Can you work these out from the model? Positions are in its coordinate system, mm. Face numbers are marked on the shaded views. A direction names the side the tool comes from. Give positions to 0.01 mm unless a question says otherwise; leave off trailing zeros. Order: outer loops, then holes, each group sorted by start corner. A loop starts at its lowest first (then second) coordinate and runs counter-clockwise, first axis right, second up. Notation, with made-up numbers: (66, -38.5) -> (91, -38.5) arc R20 cw to (91, -28.5) -> close; hole circle Ø8 at (22, 63). An arc over 180 degrees is marked (long way). Answer as a JSON object with one key per item and string values.
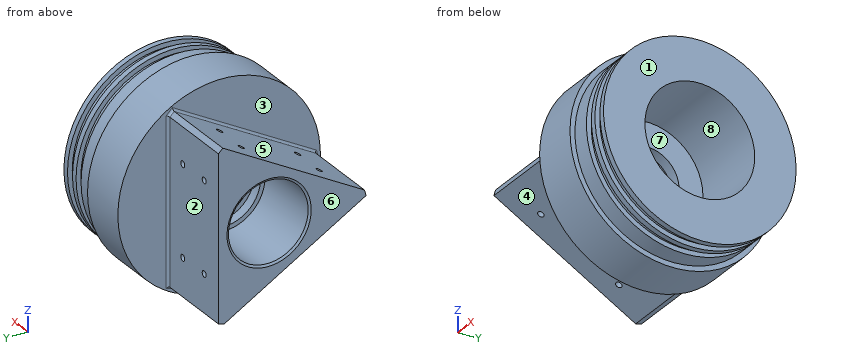
```python
from build123d import *
from OCP.BRepFilletAPI import BRepFilletAPI_MakeChamfer

# Parameters (mm, degrees)
BOSS_EXTRUDE1_DEPTH            = 22.225
SKETCH4_R                      = 22.5
CUT_EXTRUDE2_DEPTH             = 39
CHAMFER1_SIZE                  = 1.27
CHAMFER1_SIZE2                 = 0.733234842
SKETCH5_R                      = 20
CUT_EXTRUDE3_DEPTH             = 22.225
F_6_32_TAPPED_HOLE2_AT_2_COUNT = 2
F_6_32_TAPPED_HOLE2_AT_2_PITCH = 19.05
F_6_32_TAPPED_HOLE2_AT_3_COUNT = 2
F_6_32_TAPPED_HOLE2_AT_3_PITCH = 54.254423783
F_6_32_TAPPED_HOLE2_AT_4_COUNT = 2
F_6_32_TAPPED_HOLE2_AT_4_PITCH = 50.8
CIRPATTERN1_COUNT              = 3
SKETCH9_R                      = 31
CUT_EXTRUDE5_DEPTH             = 46
CUT_EXTRUDE6_REACH             = 97.461
SKETCH10_R                     = 17.5
CHAMFER2_SIZE                  = 3.81
CHAMFER2_SIZE2                 = 2.789113577
FILLET4_R                      = 1.27


with BuildPart() as part:
    # Sketch1 → Boss-Extrude1 (new, symmetric)
    with BuildSketch(Plane(origin=(0, 0, 0), x_dir=(0, 0, -1), z_dir=(1, 0, 0))):
        Polygon((-49.493351826, 28.575), (49.493351826, 28.575), (0, -57.15), align=None)
    extrude(amount=BOSS_EXTRUDE1_DEPTH, both=True)

    # Sketch4 → Cut-Extrude2 (cut)
    with BuildSketch(Plane.ZY.offset(22.225)):
        Circle(SKETCH4_R)
    extrude(amount=-CUT_EXTRUDE2_DEPTH, mode=Mode.SUBTRACT)

    # Chamfer1
    chamfer1_edges = [part.edges().sort_by_distance(p)[0] for p in [
        (-22.225, 0, -22.5),
    ]]
    chamfer1_side = [part.faces().sort_by_distance(p)[0] for p in [
        (-22.225, 27.265528995, 0),
    ]]
    chamfer(chamfer1_edges, length=CHAMFER1_SIZE, length2=CHAMFER1_SIZE2, reference=chamfer1_side[0])

    # Sketch5 → Cut-Extrude3 (cut)
    with BuildSketch(Plane(origin=(0, 0, 0), x_dir=(0, 0, -1), z_dir=(1, 0, 0))):
        with Locations(Location((0, 0, 0), (0, 0, 180))):
            Circle(SKETCH5_R)
    extrude(amount=CUT_EXTRUDE3_DEPTH, mode=Mode.SUBTRACT)

    # Sketch6 → Revolve1 (revolve)
    with BuildSketch(Plane.XY):
        Polygon((22.225, 0), (22.225, 57.15), (49.175, 57.15), (49.175, 54.3433), (59.335, 54.3433), (59.335, 51.6636), (63.78, 51.6636), (63.78, 54.3433), (66.955, 54.3433), (66.955, 51.6636), (71.4, 51.6636), (71.4, 54.3433), (74.575, 54.3433), (74.575, 0), align=None)
    revolve(axis=Axis((74.575, 0, 0), (-1, 0, 0)))

    # Sketch8 → #6-32 Tapped Hole2 (revolve, cut)
    with BuildSketch(Plane(origin=(-9.525, 28.575, -25.4), x_dir=(0, 0, 1), z_dir=(1, 0, 0))):
        Polygon((0, 0), (0, 13.51269403), (1.35255, 12.7), (1.35255, 5.588), (1.7526, 5.588), (1.7526, 0), align=None)
    f_6_32_tapped_hole2 = revolve(axis=Axis((-9.525, 34.925, -25.4), (0, -1, 0)), mode=Mode.SUBTRACT)

    # #6-32 Tapped Hole2 at 2: #6-32 Tapped Hole2 ×2
    with Locations(*[(i * F_6_32_TAPPED_HOLE2_AT_2_PITCH, 0, 0) for i in range(1, F_6_32_TAPPED_HOLE2_AT_2_COUNT)]):
        add(f_6_32_tapped_hole2, mode=Mode.SUBTRACT)

    # #6-32 Tapped Hole2 at 3: #6-32 Tapped Hole2 ×2
    with Locations(*[Vector(0.35112344158839176, 0, 0.9363291775690445) * (i * F_6_32_TAPPED_HOLE2_AT_3_PITCH) for i in range(1, F_6_32_TAPPED_HOLE2_AT_3_COUNT)]):
        add(f_6_32_tapped_hole2, mode=Mode.SUBTRACT)

    # #6-32 Tapped Hole2 at 4: #6-32 Tapped Hole2 ×2
    with Locations(*[(0, 0, i * F_6_32_TAPPED_HOLE2_AT_4_PITCH) for i in range(1, F_6_32_TAPPED_HOLE2_AT_4_COUNT)]):
        add(f_6_32_tapped_hole2, mode=Mode.SUBTRACT)

    # CirPattern1: #6-32 Tapped Hole2 ×3 about axis
    cirpattern1_axis = Axis((0, 0, 0), (1, 0, 0))
    for i in range(1, CIRPATTERN1_COUNT):
        add(f_6_32_tapped_hole2.rotate(cirpattern1_axis, i * 360 / CIRPATTERN1_COUNT), mode=Mode.SUBTRACT)

    # CirPattern1 copy 1 sketch → CirPattern1 copy 1 (revolve, cut)
    with BuildSketch(Plane(origin=(9.525, 7.709545256, 37.446675913), x_dir=(0, -0.8660254037844387, -0.4999999999999998), z_dir=(1, 0, 0))):
        Polygon((0, 0), (0, 13.51269403), (1.35255, 12.7), (1.35255, 5.588), (1.7526, 5.588), (1.7526, 0), align=None)
    revolve(axis=Axis((9.525, 4.534545256, 42.945937227), (0, 0.4999999999999998, -0.8660254037844387)), mode=Mode.SUBTRACT)

    # CirPattern1 copy 2 sketch → CirPattern1 copy 2 (revolve, cut)
    with BuildSketch(Plane(origin=(9.525, -36.284545256, -12.046675913), x_dir=(0, 0.8660254037844384, -0.5000000000000004), z_dir=(1, 0, 0))):
        Polygon((0, 0), (0, 13.51269403), (1.35255, 12.7), (1.35255, 5.588), (1.7526, 5.588), (1.7526, 0), align=None)
    revolve(axis=Axis((9.525, -39.459545256, -17.545937227), (0, 0.5000000000000004, 0.8660254037844384)), mode=Mode.SUBTRACT)

    # CirPattern1 copy 3 sketch → CirPattern1 copy 3 (revolve, cut)
    with BuildSketch(Plane(origin=(9.525, -36.284545256, 12.046675913), x_dir=(0, -0.8660254037844387, -0.4999999999999998), z_dir=(1, 0, 0))):
        Polygon((0, 0), (0, 13.51269403), (1.35255, 12.7), (1.35255, 5.588), (1.7526, 5.588), (1.7526, 0), align=None)
    revolve(axis=Axis((9.525, -39.459545256, 17.545937227), (0, 0.4999999999999998, -0.8660254037844387)), mode=Mode.SUBTRACT)

    # CirPattern1 copy 4 sketch → CirPattern1 copy 4 (revolve, cut)
    with BuildSketch(Plane(origin=(9.525, 7.709545256, -37.446675913), x_dir=(0, 0.8660254037844384, -0.5000000000000004), z_dir=(1, 0, 0))):
        Polygon((0, 0), (0, 13.51269403), (1.35255, 12.7), (1.35255, 5.588), (1.7526, 5.588), (1.7526, 0), align=None)
    revolve(axis=Axis((9.525, 4.534545256, -42.945937227), (0, 0.5000000000000004, 0.8660254037844384)), mode=Mode.SUBTRACT)

    # CirPattern1 copy 5 sketch → CirPattern1 copy 5 (revolve, cut)
    with BuildSketch(Plane(origin=(-9.525, -36.284545256, 12.046675913), x_dir=(0, -0.8660254037844387, -0.4999999999999998), z_dir=(1, 0, 0))):
        Polygon((0, 0), (0, 13.51269403), (1.35255, 12.7), (1.35255, 5.588), (1.7526, 5.588), (1.7526, 0), align=None)
    revolve(axis=Axis((-9.525, -39.459545256, 17.545937227), (0, 0.4999999999999998, -0.8660254037844387)), mode=Mode.SUBTRACT)

    # CirPattern1 copy 6 sketch → CirPattern1 copy 6 (revolve, cut)
    with BuildSketch(Plane(origin=(-9.525, 7.709545256, -37.446675913), x_dir=(0, 0.8660254037844384, -0.5000000000000004), z_dir=(1, 0, 0))):
        Polygon((0, 0), (0, 13.51269403), (1.35255, 12.7), (1.35255, 5.588), (1.7526, 5.588), (1.7526, 0), align=None)
    revolve(axis=Axis((-9.525, 4.534545256, -42.945937227), (0, 0.5000000000000004, 0.8660254037844384)), mode=Mode.SUBTRACT)

    # Sketch9 → Cut-Extrude5 (cut)
    with BuildSketch(Plane(origin=(74.575, 0, 0), x_dir=(0, 0, -1), z_dir=(1, 0, 0))):
        with Locations(Location((0, 0, 0), (0, 0, 90))):
            Circle(SKETCH9_R)
    extrude(amount=-CUT_EXTRUDE5_DEPTH, mode=Mode.SUBTRACT)

    # Sketch10 → Cut-Extrude6 (cut, up to next)
    with BuildSketch(Plane(origin=(28.575, 0, 0), x_dir=(0, 0, -1), z_dir=(1, 0, 0)), mode=Mode.PRIVATE) as cut_extrude6_sk1:
        with Locations(Location((0, 0, 0), (0, 0, 90))):
            Circle(SKETCH10_R)
    cut_extrude6_tool1 = extrude(cut_extrude6_sk1.sketch, amount=-CUT_EXTRUDE6_REACH, mode=Mode.PRIVATE) & part.part
    add(cut_extrude6_tool1.solids().sort_by_distance((28.575, 0, 0))[0], mode=Mode.SUBTRACT)

    # Chamfer2: one chamfer whose edges measure the first distance from different faces: ONE call of the kernel's chamfer builder (chamfer() names one face for all edges)
    chamfer2_edges_1 = [part.edges().sort_by_distance(p)[0] for p in [
        (0, 28.575, 49.493351826),
    ]]
    chamfer2_side_1 = [part.faces().sort_by_distance(p)[0] for p in [
        (0, 28.575, 0),
    ]]
    chamfer2_edges_2 = [part.edges().sort_by_distance(p)[0] for p in [
        (0, 28.575, -49.493351826),
    ]]
    chamfer2_side_2 = [part.faces().sort_by_distance(p)[0] for p in [
        (0, -14.2875, -24.746675913),
    ]]
    chamfer2_edges_3 = [part.edges().sort_by_distance(p)[0] for p in [
        (0, -57.15, 0),
    ]]
    chamfer2_side_3 = [part.faces().sort_by_distance(p)[0] for p in [
        (0, -14.2875, 24.746675913),
    ]]
    chamfer2 = BRepFilletAPI_MakeChamfer(part.part.solid().wrapped)
    for e in chamfer2_edges_1:
        chamfer2.Add(CHAMFER2_SIZE, CHAMFER2_SIZE2, e.wrapped, chamfer2_side_1[0].wrapped)  # the first distance lies on this face
    for e in chamfer2_edges_2:
        chamfer2.Add(CHAMFER2_SIZE, CHAMFER2_SIZE2, e.wrapped, chamfer2_side_2[0].wrapped)  # the first distance lies on this face
    for e in chamfer2_edges_3:
        chamfer2.Add(CHAMFER2_SIZE, CHAMFER2_SIZE2, e.wrapped, chamfer2_side_3[0].wrapped)  # the first distance lies on this face
    add(Compound.cast(chamfer2.Shape()), mode=Mode.REPLACE)

    # Fillet4
    fillet4_edges = [part.edges().sort_by_distance(p)[0] for p in [
        (22.225, -14.729556788, -24.491454307),
        (22.225, -13.845443212, 25.001897519),
        (22.225, 28.575, -0.510443212),
        (22.225, -54.2925, 0.255221606),
        (22.225, 26.925221606, -47.146295038),
        (22.225, 27.367278394, 46.891073432),
    ]]
    fillet(fillet4_edges, radius=FILLET4_R)


solid = part.part
```
1. Please list where these lines run through material, in increasing order: L1, parallel to X at y = -28, z = -46.5 (3 decimals); L2, parallel to X at y = 26.85, z = 25.4 (3 decimals); L3, parallel to Z at x = 46, y = 0.
Worked answers:
{"L1": "22.225 to 59.335, 63.78 to 66.955, 71.4 to 74.575", "L2": "-22.225 to -11.278, -7.772 to 7.772, 11.278 to 74.575", "L3": "-57.15 to -31, 31 to 57.15"}
2. Will these pins go through, and if not, where does the flat tip stop? pin 1 Ø2 at (x, y) = (52.5, -43) entering from -Z; pin 2 Ø1.5 at (x, y) = (55, -14) entering from -Z; pin 3 Ø8 at (x, y) = (52.5, 35.5) entering from -Z.
Worked answers:
{"pin 1": "z = -34.48", "pin 2": "z = -52.7", "pin 3": "z = -46.46"}
3. If we section it at B-B on x = -1: Please give me the cut outline in (y, z) (3 decimals).
Worked answers:
{"outline": "(-54.735, -1.395) -> (25.275, -47.588) -> (28.575, -46.704) -> (28.575, 45.683) -> (26.16, 48.099) -> (-53.85, 1.905) -> close; hole circle Ø45 at (0, 0)"}
4. If we section it at A-A on x = 18.5: Please give me the cut outline in (y, z) (3 decimals), then the cut area to 3 significant figures.
Worked answers:
{"outline": "(-54.735, -1.395) -> (25.275, -47.588) -> (28.575, -46.704) -> (28.575, 45.683) -> (26.16, 48.099) -> (-53.85, 1.905) -> close; hole circle Ø40 at (0, 0)", "area": "2,970 mm²"}
5. If we section it at C-C on x = 42: Please give me the cut outline in (y, z), then the cut area to 3 significant figures.
Worked answers:
{"outline": "circle Ø114.3 at (0, 0); hole circle Ø62 at (0, 0)", "area": "7,240 mm²"}
6. For the marked faces 1, 2, 3 and 4, which set-ups out of +Z, -Z, +X, -X, +Y, -Y let a thin tool reach every point of the face, with its end or its side?
Worked answers:
{"face 1": "+Z, -Z, +X, +Y, -Y", "face 2": "+Z, -Z, -X, +Y", "face 3": "-X", "face 4": "-Z, -X, -Y"}
7. If we mould it in two halves opening along Z, with no side actions, what happens to the marked faces 5, 6, 7 and 8? For each: +Z half, -Z half, draft (parallel to the pull), parting line (faces both ways), or undercut.
Worked answers:
{"face 5": "+Z half", "face 6": "draft", "face 7": "undercut", "face 8": "undercut"}
